Autodesk Inventor part; units mm, degrees
ref_plane "YZ Plane" through (0, 0, 0) normal (1, 0, 0) x (0, 1, 0)
ref_plane "XZ Plane" through (0, 0, 0) normal (0, 1, 0) x (-1, 0, 0)
ref_plane "XY Plane" through (0, 0, 0) normal (0, 0, 1) x (1, 0, 0)
sketch "Sketch1" plane through (0, 0, 0) normal (0, 1, 0) x (-1, 0, 0)
  line L0 (5, 0) -> (95.5, 0)
  line L1 (100.5, 5) -> (100.5, 155.5)
  line L2 (95.5, 160.5) -> (5, 160.5)
  line L3 (0, 155.5) -> (0, 5)
  arc A0 (100.5, 155.5) -> (95.5, 160.5) centre (95.5, 155.5) ccw
  arc A1 (95.5, 0) -> (100.5, 5) centre (95.5, 5) ccw
  arc A2 (0, 5) -> (5, 0) centre (5, 5) ccw
  arc A3 (5, 160.5) -> (0, 155.5) centre (5, 155.5) ccw
  line L4 (105.5, 155.5) -> (105.5, 5)
  arc A4 (95.5, -5) -> (105.5, 5) centre (95.5, 5) ccw
  line L5 (95.5, -5) -> (5, -5)
  arc A5 (-5, 5) -> (5, -5) centre (5, 5) ccw
  line L6 (-5, 5) -> (-5, 155.5)
  arc A6 (5, 165.5) -> (-5, 155.5) centre (5, 155.5) ccw
  line L7 (5, 165.5) -> (95.5, 165.5)
  arc A7 (105.5, 155.5) -> (95.5, 165.5) centre (95.5, 155.5) ccw
  point P0 (0, 0)
  point P1 (100.5, 160.5)
  point P2 (100.5, 0)
  point P3 (0, 160.5)
  dimension "d0" = 100.5
  dimension "d1" = 160.5
  dimension "d2" = 5
  dimension "d3" = 5
extrude "Extrusion1" add sketch "Sketch1" along normal blind 4
sketch "Sketch2" plane through (0, 0, 0) normal (0, -1, 0) x (1, 0, 0)
  line L0 (5, 155.5) -> (5, 5)
  arc A0 (5, 155.5) -> (-5, 165.5) centre (-5, 155.5) ccw
  line L1 (-95.5, 165.5) -> (-5, 165.5)
  arc A1 (-95.5, 165.5) -> (-105.5, 155.5) centre (-95.5, 155.5) ccw
  line L2 (-105.5, 5) -> (-105.5, 155.5)
  arc A2 (-105.5, 5) -> (-95.5, -5) centre (-95.5, 5) ccw
  line L3 (-5, -5) -> (-95.5, -5)
  arc A3 (-5, -5) -> (5, 5) centre (-5, 5) ccw
  arc A4 (-5, 0) -> (0, 5) centre (-5, 5) ccw
  line L4 (-95.5, 0) -> (-5, 0)
  arc A5 (-100.5, 5) -> (-95.5, 0) centre (-95.5, 5) ccw
  line L5 (-100.5, 155.5) -> (-100.5, 5)
  arc A6 (-95.5, 160.5) -> (-100.5, 155.5) centre (-95.5, 155.5) ccw
  line L6 (-5, 160.5) -> (-95.5, 160.5)
  arc A7 (0, 155.5) -> (-5, 160.5) centre (-5, 155.5) ccw
  line L7 (0, 5) -> (0, 155.5)
  line L8 (14.75, 145.25) -> (-115.25, 145.25) construction
  line L9 (-115.25, 145.25) -> (-115.25, 15.25) construction
  line L10 (-115.25, 15.25) -> (14.75, 15.25) construction
  line L11 (14.75, 15.25) -> (14.75, 145.25) construction
  circle A8 centre (14.75, 145.25) radius 2.75
  arc A9 (14.75, 135.5) -> (14.75, 155) centre (14.75, 145.25) ccw
  line L12 (5, 155.5) -> (5, 5)
  line L13 (5, 155.5) -> (5, 5)
  line L14 (5, 135.5) -> (14.75, 135.5)
  line L15 (5, 155) -> (14.75, 155)
  line L16 (0, 5) -> (0, 155.5) construction
  line L17 (0, 80.25) -> (-100.5, 80.25) construction
  line L18 (-100.5, 155.5) -> (-100.5, 5) construction
  line L19 (-50.25, 80.25) -> (-50.25, 145.25) construction
  circle A10 centre (14.75, 15.25) radius 2.75
  arc A11 (14.75, 5.5) -> (14.75, 25) centre (14.75, 15.25) ccw
  line L20 (5, 25) -> (14.75, 25)
  line L21 (5, 5.5) -> (14.75, 5.5)
  circle A12 centre (-115.25, 145.25) radius 2.75
  arc A13 (-115.25, 155) -> (-115.25, 135.5) centre (-115.25, 145.25) ccw
  line L22 (-105.5, 135.5) -> (-115.25, 135.5)
  line L23 (-105.5, 155) -> (-115.25, 155)
  arc A14 (-115.25, 25) -> (-115.25, 5.5) centre (-115.25, 15.25) ccw
  line L24 (-105.5, 25) -> (-115.25, 25)
  circle A15 centre (-115.25, 15.25) radius 2.75
  line L25 (-105.5, 5.5) -> (-115.25, 5.5)
  point P0 (0, 0)
  dimension "d6" = 130
  dimension "d7" = 130
  dimension "d8" = 110.5
  dimension "d9" = 9.75
  dimension "d10" = 170.5
  dimension "d11" = 20.25
  dimension "d12" = 5.5
extrude "Extrusion2" add sketch "Sketch2" along normal blind 4 contours L0 A3 L3 A2 L2 A1 L1 A0 | L15 A9 L14 L0 | L20 A11 L21 L0 | L2 L22 A13 L23 | L2 L25 A14 L24 | L4 A5 L5 A6 L6 A7 L7 A4
sketch "Sketch3" plane through (0, 0, 0) normal (0, 1, 0) x (1, 0, 0)
  line L0 (-5.25, -155.25) -> (-95.25, -155.25) construction
  line L1 (-95.25, -155.25) -> (-95.25, -5.25) construction
  line L2 (-95.25, -5.25) -> (-5.25, -5.25) construction
  line L3 (-5.25, -5.25) -> (-5.25, -155.25) construction
  line L4 (-50.25, -155.25) -> (-50.25, -160.5) construction
  line L5 (-5, -160.5) -> (-95.5, -160.5) construction
  line L6 (-5.25, -80.25) -> (0, -80.25) construction
  line L7 (-50.25, -5.25) -> (-50.25, 0) construction
  line L8 (-95.5, 0) -> (-5, 0) construction
  line L9 (-95.25, -80.25) -> (-100.5, -80.25) construction
  line L10 (-100.5, -155.5) -> (-100.5, -5) construction
  line L11 (0, -5) -> (0, -155.5)
  line L12 (-100.5, -155.5) -> (-100.5, -5)
  arc A0 (-5, -160.5) -> (0, -155.5) centre (-5, -155.5) ccw
  arc A1 (-100.5, -155.5) -> (-95.5, -160.5) centre (-95.5, -155.5) ccw
  circle A2 centre (-5.25, -5.25) radius 3.5
  circle A3 centre (-5.25, -155.25) radius 3.5
  circle A4 centre (-95.25, -155.25) radius 3.5
  circle A5 centre (-95.25, -5.25) radius 3.5
  point P0 (0, 0)
  dimension "d15" = 90
  dimension "d16" = 150
  dimension "d17" = 7
  dimension "d18" = 7
  dimension "d19" = 7
  dimension "d20" = 7
extrude "Extrusion3" add sketch "Sketch3" along normal blind 2.3
sketch "Sketch4" plane through (-95.25, 2.3, 155.25) normal (0, 1, 0) x (1, 0, 0)
  circle A0 centre (90, 0) radius 3.5
  circle A1 centre (0, 0) radius 3.5
  circle A2 centre (90, 150) radius 3.5
  circle A3 centre (0, 150) radius 3.5
  circle A4 centre (90, 0) radius 1.5
  circle A5 centre (0, 0) radius 3.5
  circle A6 centre (0, 0) radius 1.5
  circle A7 centre (90, 150) radius 3.5
  circle A8 centre (90, 150) radius 1.5
  circle A9 centre (0, 150) radius 1.5
  point P0 (95.25, 155.25)
  dimension "d23" = 3
  dimension "d24" = 3
  dimension "d25" = 3
  dimension "d26" = 3
extrude "Extrusion4" cut sketch "Sketch4" against normal through all contours A4 | A6 | A8 | A9
chamfer "Chamfer1" distance 1 angle 45 4 edges at (-96.75, 2.3, 155.25) (-6.75, 2.3, 155.25) (-6.75, 2.3, 5.25) (-96.75, 2.3, 5.25)
chamfer "Chamfer2" distance 1 angle 45 4 edges at (-98.75, 0, 155.25) (-8.75, 0, 155.25) (-98.75, 0, 5.25) (-8.75, 0, 5.25)
equation "\"d9\" = -0.5 * d8 + 0.5 * d6"
equation "\"d11\" = -0.5 * d7 + 0.5 * d10"
equation "\"d18\" = d17"
equation "\"d19\" = d17"
equation "\"d20\" = d17"
equation "\"d24\" = d23"
equation "\"d25\" = d23"
equation "\"d26\" = d23"
properties part number "BTT Octopus 1.1 Mount"
Geometry: final body of the model. Coordinates: model frame, mm. A direction names the side the tool comes from. Give positions to 0.01 mm unless a question says otherwise; leave off trailing zeros. Order: outer loops, then holes, each group sorted by start corner. A loop starts at its lowest first (then second) coordinate and runs counter-clockwise, first axis right, second up. Notation, with made-up numbers: M -33.75,-22 L -29.75,-22 A18 cw -29.75,-18 Z; hole C 78.5,-18 d9. An arc over 180 degrees is marked long. Answer as CSV lines item,"result". Start each with the question number.
1) Set-up query: faces 4 (the flat face through (-110, -2, 5.5)), 5 (the flat face through (-113, 0, 13)), 6 (the flat face through (10, -2, 25)), 7 (the cylindrical face through (-2, 2, 1)), 8 (the flat face through (10, -2, 5.5)). Return all of +Z, -Z, +X, -X, +Y, -Y with unobstructed straight access to the full face (end or side cutting, diameter ignored); none if empty.
2) First-contact query: P1, Ø5.5, axis at x = -4, z = 155, coming from the +Y side; P2, Ø4.5, axis at x = 8.5, y = -1.5, coming from the +Z side; P3, Ø6, axis at x = -5.5, z = 81, coming from the +Y side; P4, Ø4.5, axis at x = 14.75, z = 145.25, coming from the -Y side. Flat tips, straight axial feed; report the tip coordinate or a pass-through.
3) Cut plane A-A (x = 10). Output: boundary loops of the cut face in (y, z), then the cut area to 3 significant figures.
4) Cut plane B-B (z = 15.25). Output: boundary loops of the cut face in (x, y).
5) Cut plane C-C (z = 115). Output: boundary loops of the cut face in (x, y), then the cut area to 3 significant figures.
6) Mould query, pull axis Z, two halves, no side actions, for faces 1 (the cylindrical face through (1.99, -0.06, -2.15)), 2 (the flat face through (-50, 0, 165.5)), 3 (the flat face through (-110, -2, 25)). Classes: +Z half, -Z half, draft (parallel to the pull), parting line (faces both ways), or undercut.
7) Line query: line 1 (Z direction, x = -95.25, y = -0.55); line 2 (Z direction, x = 14.75, y = -2.05); line 3 (X direction, y = -1.8, z = 145.25). Output: solid intervals per line, ascending. Write a range as from..to.
8) Cut plane D-D (x = -27.5). Output: boundary loops of the cut face in (y, z), then the cut area to 3 significant figures.
Findings below:
1,face 4,"-Z, -X, +Y, -Y"
1,face 5,"+Z, -Z, -X, +Y"
1,face 6,"+X, +Y, -Y"
1,face 7,"+Y"
1,face 8,"-Z, +X, +Y, -Y"
2,P1,"stops at y = 2.3"
2,P2,"stops at z = 155"
2,P3,"stops at y = 0"
2,P4,"passes through"
3,outline,"M -4,5.5 L 0,5.5 L 0,25 L -4,25 Z; M -4,135.5 L 0,135.5 L 0,155 L -4,155 Z"
3,area,"156 mm²"
4,outline,"M -125,-4 L -118,-4 L -118,0 L -125,0 Z; M -112.5,-4 L 12,-4 L 12,0 L 5,0 L 5,4 L 0,4 L 0,0 L -100.5,0 L -100.5,4 L -105.5,4 L -105.5,0 L -112.5,0 Z; M 17.5,-4 L 24.5,-4 L 24.5,0 L 17.5,0 Z"
5,outline,"M -105.5,-4 L 5,-4 L 5,4 L 0,4 L 0,0 L -100.5,0 L -100.5,4 L -105.5,4 Z"
5,area,"482 mm²"
6,face 1,"-Z half"
6,face 2,"+Z half"
6,face 3,"undercut"
7,line 1,"z = -5..3.75, 6.75..153.75, 156.75..165.5"
7,line 2,"z = 5.5..12.5, 18..25, 135.5..142.5, 148..155"
7,line 3,"x = -125..-118, -112.5..12, 17.5..24.5"
8,outline,"M -4,-5 L 4,-5 L 4,0 L 0,0 L 0,160.5 L 4,160.5 L 4,165.5 L -4,165.5 Z"
8,area,"722 mm²"
